```python
from build123d import *

# Parameters (mm, degrees)
SKETCH_1_W           = 30
SKETCH_1_H           = 50
EXTRUDE_1_DEPTH      = 5
SKETCH_5_W           = 30
SKETCH_5_H           = 50
EXTRUDE_2_DEPTH      = 4.5
SKETCH_6_R           = 1.5
CUT_EXTRUDE_1_DEPTH  = 73.857738093
SKETCH_7_R           = 1.5
CUT_EXTRUDE_2_DEPTH  = 73.857738093
SKETCH_12_W          = 12.5
SKETCH_12_H          = 10
CUT_EXTRUDE_8_DEPTH  = 71.551399703
SKETCH_13_W          = 12.5
SKETCH_13_H          = 10
CUT_EXTRUDE_9_DEPTH  = 71.551399703
SKETCH_16_W          = 30
SKETCH_16_H          = 5
EXTRUDE_3_DEPTH      = 20
SKETCH_17_R          = 1.5
CUT_EXTRUDE_10_DEPTH = 20
SKETCH_18_W          = 53.118549685
SKETCH_18_H          = 48.988218424
CUT_EXTRUDE_11_DEPTH = 20
FILLET_1_R           = 2
FILLET_2_R           = 2
FILLET_3_R           = 2
FILLET_4_R           = 2
SKETCH_19_R          = 1.5
CUT_EXTRUDE_12_DEPTH = 10
SKETCH_21_R          = 1.5
EXTRUDE_4_DEPTH      = 5


with BuildPart() as part:
    # 草图1 → 凸台-拉伸1 (new body)
    with BuildSketch(Plane.XY):
        Rectangle(SKETCH_1_W, SKETCH_1_H)
    extrude(amount=EXTRUDE_1_DEPTH)

    # 草图5 → 凸台-拉伸2 (add)
    with BuildSketch(Plane.ZY.offset(15)):
        with Locations((2.5, 34)):
            Rectangle(SKETCH_5_W, SKETCH_5_H)
    extrude_2 = extrude(amount=EXTRUDE_2_DEPTH)

    # 镜向1: 凸台-拉伸2 across plane
    add(extrude_2.mirror(Plane(origin=(0, 0, 0), x_dir=(0, 0, 1), z_dir=(1, 0, 0))))

    # 草图6 → 切除-拉伸1 (cut, through all)
    with BuildSketch(Plane.ZY.offset(19.5)):
        with Locations((2.5, 55)):
            Circle(SKETCH_6_R)
    extrude(amount=-CUT_EXTRUDE_1_DEPTH, mode=Mode.SUBTRACT)

    # 草图7 → 切除-拉伸2 (cut, through all)
    with BuildSketch(Plane.ZY.offset(19.5)):
        with Locations((-7.5, 55)):
            Circle(SKETCH_7_R)
        with Locations((12.5, 55)):
            Circle(SKETCH_7_R)
    extrude(amount=-CUT_EXTRUDE_2_DEPTH, mode=Mode.SUBTRACT)

    # 草图12 → 切除-拉伸8 (cut, through all)
    with BuildSketch(Plane(origin=(-15, 0, 0), x_dir=(0, 0, -1), z_dir=(1, 0, 0))):
        with Locations((6.25, 14)):
            Rectangle(SKETCH_12_W, SKETCH_12_H)
        with Locations((-11.25, 14)):
            Rectangle(SKETCH_12_W, SKETCH_12_H)
    extrude(amount=-CUT_EXTRUDE_8_DEPTH, mode=Mode.SUBTRACT)

    # 草图13 → 切除-拉伸9 (cut, through all)
    with BuildSketch(Plane.ZY.offset(-15)):
        with Locations((11.25, 14)):
            Rectangle(SKETCH_13_W, SKETCH_13_H)
        with Locations((-6.25, 14)):
            Rectangle(SKETCH_13_W, SKETCH_13_H)
    extrude(amount=-CUT_EXTRUDE_9_DEPTH, mode=Mode.SUBTRACT)

    # 草图16 → 凸台-拉伸3 (add)
    with BuildSketch(Plane(origin=(0, 25, 0), x_dir=(1, 0, 0), z_dir=(0, 1, 0))):
        with Locations((0, -2.5)):
            Rectangle(SKETCH_16_W, SKETCH_16_H)
    extrude(amount=EXTRUDE_3_DEPTH)

    # 草图17 → 切除-拉伸10 (cut)
    with BuildSketch(Plane.XY.offset(5)):
        with Locations((0, 12.5)):
            Circle(SKETCH_17_R)
    extrude(amount=-CUT_EXTRUDE_10_DEPTH, mode=Mode.SUBTRACT)

    # 草图18 → 切除-拉伸11 (cut)
    with BuildSketch(Plane.XY.offset(5)):
        with Locations((5.810767558, -19.494109212)):
            Rectangle(SKETCH_18_W, SKETCH_18_H)
    extrude(amount=-CUT_EXTRUDE_11_DEPTH, mode=Mode.SUBTRACT)

    # 圆角1
    fillet_1_edges = [part.edges().sort_by_distance(p)[0] for p in [
        (17.25, 19, 5),
        (17.25, 19, 0),
        (-17.25, 19, 0),
        (-17.25, 19, 5),
    ]]
    fillet(fillet_1_edges, radius=FILLET_1_R)

    # 圆角2
    fillet_2_edges = [part.edges().sort_by_distance(p)[0] for p in [
        (15, 31, 0),
        (-15, 31, 0),
        (15, 31, 5),
        (-15, 31, 5),
    ]]
    fillet(fillet_2_edges, radius=FILLET_2_R)

    # 圆角3
    fillet_3_edges = [part.edges().sort_by_distance(p)[0] for p in [
        (17.25, 19, 17.5),
        (17.25, 19, -12.5),
        (-17.25, 59, -12.5),
        (-17.25, 59, 17.5),
        (17.25, 59, -12.5),
        (17.25, 59, 17.5),
        (-17.25, 19, -12.5),
        (-17.25, 19, 17.5),
    ]]
    fillet(fillet_3_edges, radius=FILLET_3_R)

    # 圆角4
    fillet_4_edges = [part.edges().sort_by_distance(p)[0] for p in [
        (15, 9, 2.5),
        (-15, 9, 2.5),
        (19.5, 9, 2.5),
        (15, 5, 2.5),
        (-15, 5, 2.5),
        (-19.5, 9, 2.5),
    ]]
    fillet(fillet_4_edges, radius=FILLET_4_R - 0.0001)  # a hair under: the kernel refuses the full size

    # 草图19 → 切除-拉伸12 (cut)
    with BuildSketch(Plane.XY.offset(5)):
        with Locations((0, 17.5)):
            Circle(SKETCH_19_R)
    extrude(amount=-CUT_EXTRUDE_12_DEPTH, mode=Mode.SUBTRACT)

    # 草图21 → 凸台-拉伸4 (add)
    with BuildSketch(Plane.XY.offset(5)):
        with Locations((0, 12.5)):
            Circle(SKETCH_21_R)
    extrude(amount=-EXTRUDE_4_DEPTH)


solid = part.part
```
For this review, take the finished solid that the model builds, in its own axes (mm). A direction names the side the tool comes from. Round coordinates to 2 decimals unless told otherwise and drop trailing zeros. Write each loop counter-clockwise with the first axis right and the second up, starting at its lowest first coordinate (ties: lowest second). Pieces come first, ordered by that corner, then holes. Notation, with made-up numbers: (-20.5, -39) -> (-12.5, -39) arc R22 ccw to (-12.5, -3) -> close; hole circle Ø10 at (74.5, 70.5). An arc over 180 degrees is marked (long way). Use one line per item in the form item = value.
Q1. Machinability: for faces 5 (the flat face through (-17, 19, 11)), 6 (the flat face through (-17, 19, -6)), 7 (the flat face through (0, 45, 2)), which of the approach directions +Z, -Z, +X, -X, +Y, -Y give a long, thin tool a straight path to every point of the face, cutting with its end or side? Answer none if there is none.
Resolved:
face_5 = +Z, +X, -X, -Y
face_6 = -Z, +X, -X, -Y
face_7 = +Z, -Z, +Y
Q2. To check wall thickness, follow probe 1 along Y at (x, z) = (-17, -7.5); probe 2 along Y at (x, z) = (0, 3.9); probe 3 along X at (y, z) = (27, -6). State the ranges of each line that lie inside material, in increasing order. Write a range as from..to.
Resolved:
probe_1 = 19..53.5, 56.5..59
probe_2 = 5..16, 19..45
probe_3 = -19.5..-15, 15..19.5
Q3. The part is to be moulded in two halves that separate along X. For faces 1 (the flat face through (17, 19, 11)), 2 (the cylindrical face through (14.43, 5.6, 2.54)), 3 (the flat face through (0, 25, 5)), 4 (the flat face through (0, 25, 0)), say which applies: released by +X, released by -X, zero draft, split by the parting line, or undercut.
Resolved:
face_1 = zero draft
face_2 = released by +X
face_3 = undercut
face_4 = undercut
Q4. Consider section C-C (y = 47.5). State the section outline as (x, z) points.
Resolved:
outline = (-19.5, -12.5) -> (-15, -12.5) -> (-15, 17.5) -> (-19.5, 17.5) -> close; (15, -12.5) -> (19.5, -12.5) -> (19.5, 17.5) -> (15, 17.5) -> close
Q5. Consider section D-D (z = 12.5). State the section outline as (x, y) points.
Resolved:
outline = (-19.5, 19) -> (-15, 19) -> (-15, 53.5) -> (-19.5, 53.5) -> close; (-19.5, 56.5) -> (-15, 56.5) -> (-15, 59) -> (-19.5, 59) -> close; (15, 19) -> (19.5, 19) -> (19.5, 53.5) -> (15, 53.5) -> close; (15, 56.5) -> (19.5, 56.5) -> (19.5, 59) -> (15, 59) -> close
Q6. Consider section A-A (z = 2.5). State how many separate pieces and enclosed holes the cut face has, then the cut area to 3 significant figures.
Resolved:
separate_pieces = 3
enclosed_holes = 1
area = 1,610 mm²
Q7. Clearance check with flat-ended pins moving along their axes: pin 1 Ø2.5 at (x, y) = (0, 17.5) entering from +Z; pin 2 Ø6 at (x, y) = (-12, 12.5) entering from -Z; pin 3 Ø1.3 at (x, z) = (17.5, 11) entering from -Y; pin 4 Ø10 at (x, y) = (-9.5, 29.5) entering from -Z. State where each tip first meets the part, or that it passes through.
Resolved:
pin_1 = through
pin_2 = 0
pin_3 = 19
pin_4 = -0.68
